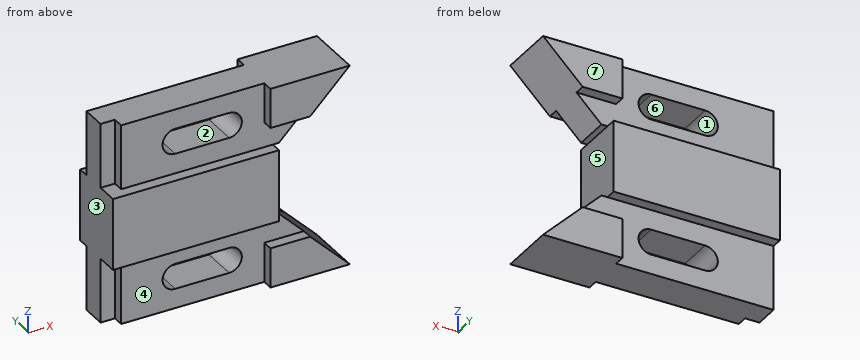
```python
from build123d import *

# Parameters (mm, degrees)
F1_DEPTH = 7.874
F2_DEPTH = 12.7
F0_W     = 73.406
F0_H     = 15.875
F3_DEPTH = 12.7
F4_W     = 6.35
F4_H     = 28.575
F5_DEPTH = 4.826


with BuildPart() as f1:
    # F0 (on Front) → F1 (new body, symmetric)
    with BuildSketch(Plane.XZ):
        Polygon((0, 44.45), (0, 15.875), (73.406, 15.875), (76.073, 15.875), (87.122, 26.924), (69.596, 26.924), (69.596, 44.45), align=None)
        with BuildLine():
            ThreePointArc((30.226, 24.638), (24.638, 30.226), (30.226, 35.814))
            Line((30.226, 35.814), (54.102, 35.814))
            ThreePointArc((54.102, 35.814), (59.69, 30.226), (54.102, 24.638))
            Line((54.102, 24.638), (30.226, 24.638))
        make_face(mode=Mode.SUBTRACT)
    extrude(amount=F1_DEPTH, both=True)

    # F0 (on Front) → F2 (join, symmetric)
    with BuildSketch(Plane.XZ):
        Polygon((104.648, 44.45), (69.596, 44.45), (69.596, 26.924), (87.122, 26.924), align=None)
    extrude(amount=F2_DEPTH, both=True)

    # F0 (on Front) → F3 (join, symmetric)
    with BuildSketch(Plane.XZ):
        with Locations((36.703, 7.9375)):
            Rectangle(F0_W, F0_H)
    extrude(amount=F3_DEPTH, both=True)

    # F4 (on face) → F5 (cut)
    with BuildSketch(Plane.XZ.offset(7.874)):
        with Locations((3.175, 30.1625)):
            Rectangle(F4_W, F4_H)
    extrude(amount=-F5_DEPTH, mode=Mode.SUBTRACT)

    # F6: F1 across plane


with BuildPart() as f1_1:
    add(f1.part)
    add(f1.part.mirror(Plane.XY))


solid = f1_1.part
```
Geometry: final body of the model. Coordinates: model frame, mm. Face numbers are marked on the shaded views. A direction names the side the tool comes from. Coordinates: 2 decimals unless noted, no trailing zeros. Order: outer loops, then holes, each group sorted by start corner. A loop starts at its lowest first (then second) coordinate and runs counter-clockwise, first axis right, second up. Notation, with made-up numbers: M -17.75,35 L 33.25,35 A8 ccw 33.25,44 Z; hole C 42.5,32 d4. An arc over 180 degrees is marked long. Answer as CSV lines item,"result".
Q1. Section C-C on y = 5. Return the cut outline in (x, z) (3 decimals), and give its area (3 significant figures).
Answers:
outline,"M 0,-44.45 L 104.648,-44.45 L 76.073,-15.875 L 73.406,-15.875 L 73.406,15.875 L 76.073,15.875 L 104.648,44.45 L 0,44.45 Z; hole M 30.226,-35.814 L 54.102,-35.814 A5.588 ccw 54.102,-24.638 L 30.226,-24.638 A5.588 ccw Z; hole M 30.226,24.638 L 54.102,24.638 A5.588 ccw 54.102,35.814 L 30.226,35.814 A5.588 ccw Z"
area,"6,760 mm^2"
Q2. Set-up query: the marked faces 5, 6 and 7. Return all of +Z, -Z, +X, -X, +Y, -Y with unobstructed straight access to the full face (end or side cutting, diameter ignored); none if empty.
Answers:
face 5,"+X, +Y, -Y"
face 6,"+Y, -Y"
face 7,"+Z, -Z, +X, -X, +Y"
Q3. Section D-D on z = -31. Return the cut outline in (x, y), and give its area (3 significant figures).
Answers:
outline,"M 0,-3.05 L 6.35,-3.05 L 6.35,-7.87 L 24.69,-7.87 L 24.69,7.87 L 0,7.87 Z; M 59.64,-7.87 L 69.6,-7.87 L 69.6,-12.7 L 91.2,-12.7 L 91.2,12.7 L 69.6,12.7 L 69.6,7.87 L 59.64,7.87 Z"
area,"1,060 mm^2"
Q4. Section A-A on y = -9.5. Return the cut outline in (x, z) (3 decimals).
Answers:
outline,"M 0,-15.875 L 73.406,-15.875 L 73.406,15.875 L 0,15.875 Z; M 69.596,-44.45 L 104.648,-44.45 L 87.122,-26.924 L 69.596,-26.924 Z; M 69.596,26.924 L 87.122,26.924 L 104.648,44.45 L 69.596,44.45 Z"
Q5. Draft query along X for the marked faces 1, 2, 3 and 4. Return one class per face: pulls with the +X half, pulls with the -X half, needs draft (parallel to the pull), parting line crosses it, or undercut.
Answers:
face 1,"undercut"
face 2,"undercut"
face 3,"pulls with the -X half"
face 4,"needs draft"
Q6. Section B-B on x = 47.5. Return the cut outline in (y, z) (3 decimals), and give its area (3 significant figures).
Answers:
outline,"M -12.7,-15.875 L -7.874,-15.875 L -7.874,-24.638 L 7.874,-24.638 L 7.874,-15.875 L 12.7,-15.875 L 12.7,15.875 L 7.874,15.875 L 7.874,24.638 L -7.874,24.638 L -7.874,15.875 L -12.7,15.875 Z; M -7.874,-44.45 L 7.874,-44.45 L 7.874,-35.814 L -7.874,-35.814 Z; M -7.874,35.814 L 7.874,35.814 L 7.874,44.45 L -7.874,44.45 Z"
area,"1,350 mm^2"
Q7. First-contact query: P1, Ø2, axis at y = 2.5, z = -14.5, coming from the -X side; P2, Ø5, axis at y = -1, z = 31, coming from the +X side; P3, Ø1.4, axis at y = -5.5, z = 30, coming from the -X side; P4, Ø1.4, axis at x = 30, y = 10.5, coming from the -Z side (3 decimals). Flat tips, straight axial feed; report the tip coordinate or a pass-through.
Answers:
P1,"stops at x = 0"
P2,"stops at x = 93.7"
P3,"stops at x = 6.35"
P4,"stops at z = -15.875"
Q8. Line query: probe 1 along Z at (x, y) = (47, 6.5); probe 2 along Z at (x, y) = (80, 9.25); probe 3 along Z at (x, y) = (28.5, 3.25). Output: solid intervals per line, ascending. Write a range as [from, to].
Answers:
probe 1,"z = [-44.45, -35.81], [-24.64, 24.64], [35.81, 44.45]"
probe 2,"z = [-44.45, -26.92], [26.92, 44.45]"
probe 3,"z = [-44.45, -35.54], [-24.91, 24.91], [35.54, 44.45]"
